Geometry: see drawing. Coordinates: mm, zero at the bounding-box minimum. A direction names the side the tool comes from. Coordinates: 2 decimals unless noted, no trailing zeros. Write each loop counter-clockwise with the first axis right and the second up, starting at its lowest first coordinate (ties: lowest second). Pieces come first, ordered by that corner, then holes. Notation, with made-up numbers: M 72,-34 L 89,-34 A16 ccw 89,-11 Z; hole C 9.25,-36.75 d9. An arc over 180 degrees is marked long. Write item = value, one per line. Start each with the question number.
1. Section query A-A (y = 3). Output: boundary loops of the cut face in (x, z).
2. Access query for the marked faces 1, 2 and 3. Directions: +Z, -Z, +X, -X, +Y, -Y. A direction counts if a zero-diameter tool reaches every point of the face in a straight line with its end or side. Return the directions, or none.
3. Pin query (flat end, axial travel): pin 1 Ø1.5 at (x, z) = (5, 12) entering from +Y; pin 2 Ø1 at (y, z) = (4.5, 2.5) entering from +X; pin 3 Ø1.5 at (y, z) = (4, 17) entering from -X. Return the tip coordinate at first contact, or that it passes through.
4. Section query D-D (z = 19.75). Output: boundary loops of the cut face in (x, y).
5. Line query: line 1 along Z through (x, y) = (5.65, 2.8); line 2 along X through (y, z) = (5.35, 9.75); line 3 along Y through (x, z) = (4.3, 10.5). Output: solid intervals per line, ascending.
6. Section query C-C (z = 10.25). Output: boundary loops of the cut face in (x, y), then the cut area to 3 significant figures.
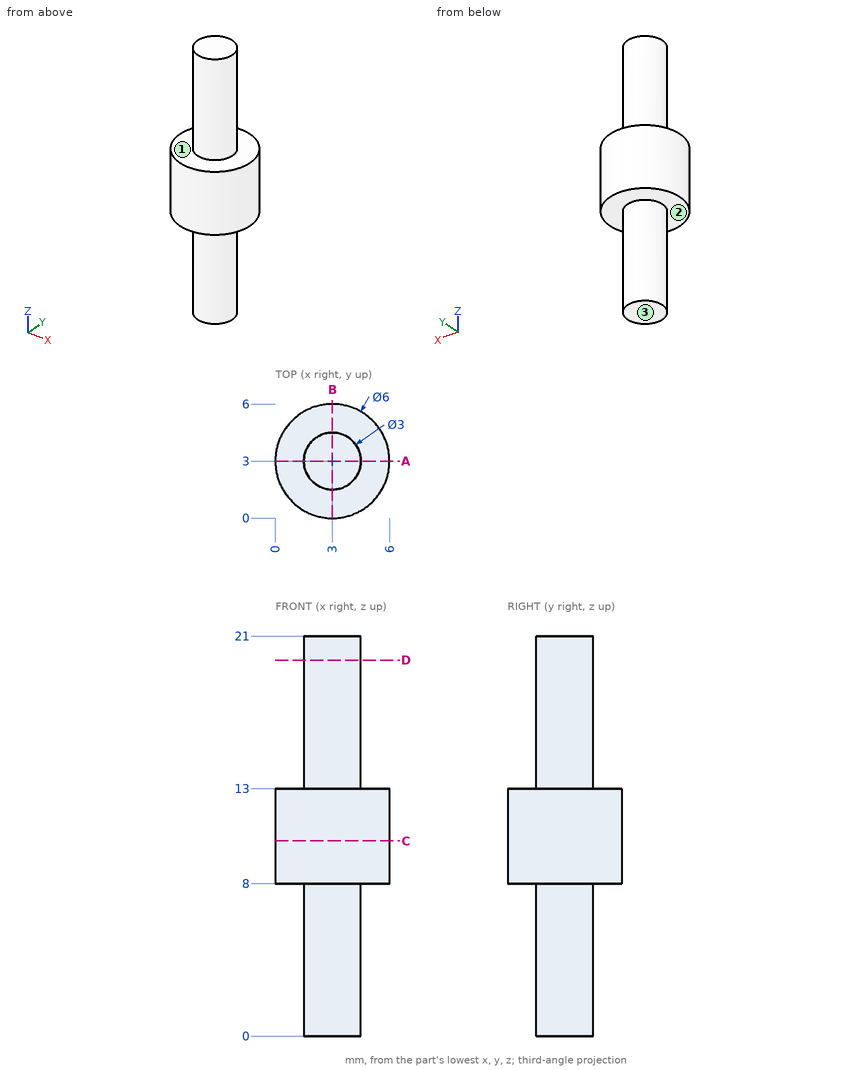
Results are:
q1.outline = M 0,8 L 1.5,8 L 1.5,0 L 4.5,0 L 4.5,8 L 6,8 L 6,13 L 4.5,13 L 4.5,21 L 1.5,21 L 1.5,13 L 0,13 Z
q2.face_1 = +Z
q2.face_2 = -Z
q2.face_3 = -Z, +X, -X, +Y, -Y
q3.pin_1 = 5.73
q3.pin_2 = 4.12
q3.pin_3 = 1.52
q4.outline = C 3,3 d3
q5.line_1 = 8 to 13
q5.line_2 = 1.14 to 4.86
q5.line_3 = 0.3 to 5.7
q6.outline = C 3,3 d6
q6.area = 28.3 mm^2
